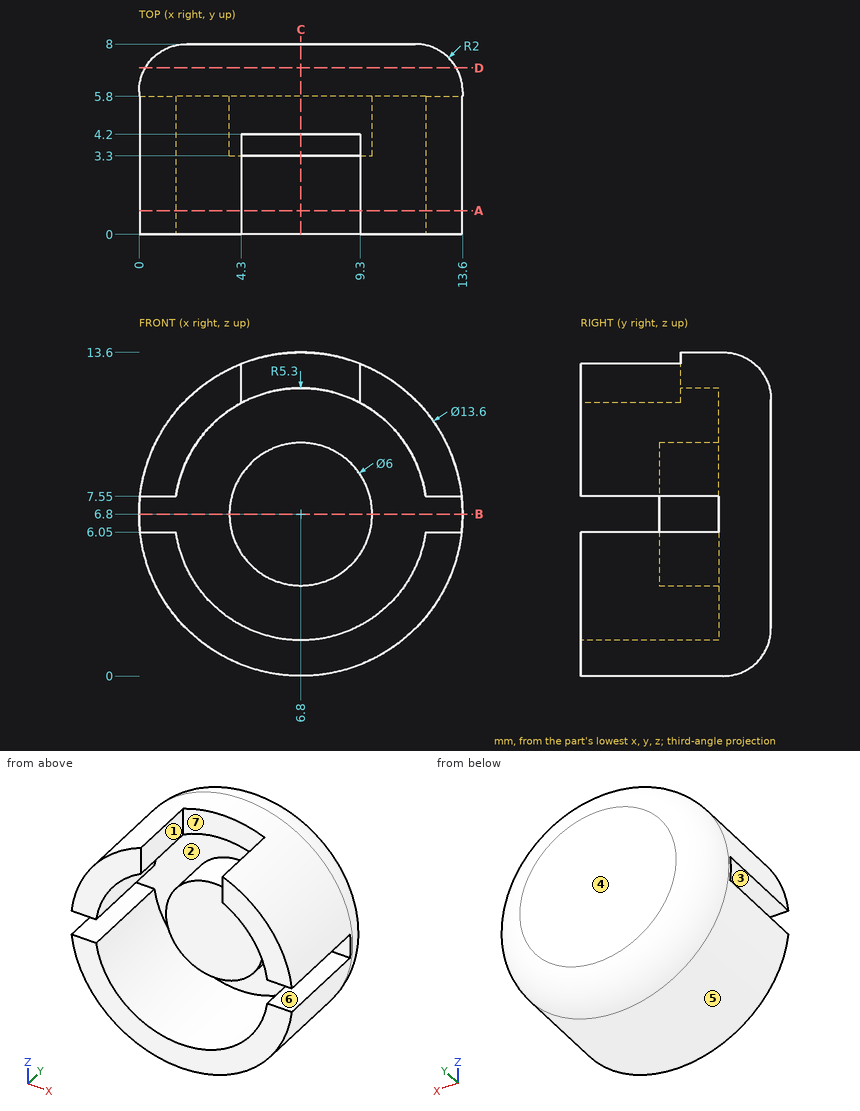
Geometry: see drawing. Coordinates: mm, zero at the bounding-box minimum. A direction names the side the tool comes from. Round coordinates to 2 decimals unless told otherwise and drop trailing zeros. Loops run counter-clockwise (first coordinate to the right, second up) from the corner with the lowest first, then second, coordinate; pieces in that order, holes last. Notation, with made-up numbers: (-32, 33.25) - (17, 33.25) arc R20 ccw to (17, 54.25) - close; hole circle Ø7 at (15, -27.5). An arc over 180 degrees is marked (long way). Use CSV: the item, a comma, the result in double quotes.
Q1. Mould query, pull axis Z, two halves, no side actions, for the marked faces 5, 6 and 7. Classes: pulls with the +Z half, pulls with the -Z half, needs draft (parallel to the pull), parting line crosses it, or undercut.
Reported:
face 5,"parting line crosses it"
face 6,"undercut"
face 7,"needs draft"
Q2. Section query D-D, the plane y = 7. Output: boundary loops of the cut face in (x, z).
Reported:
outline,"circle Ø13.06 at (6.8, 6.8)"
Q3. Reachability of the marked faces 1, 2, 3 and 4 from +Z, -Z, +X, -X, +Y, -Y: full face, straight path, thin tool, end or side. Return the list, or none.
Reported:
face 1,"+Z, -Y"
face 2,"-Y"
face 3,"-X, -Y"
face 4,"+Z, -Z, +X, -X, +Y"
Q4. Pin query (flat end, axial travel): pin 1 Ø1.2 at (x, y) = (13, 2) entering from -Z; pin 2 Ø1 at (x, y) = (2.5, 3.5) entering from -Z; pin 3 Ø0.5 at (x, y) = (0.5, 4) entering from -Z. Return the tip coordinate at first contact, or that it passes through.
Reported:
pin 1,"z = 2.94"
pin 2,"z = 1.16"
pin 3,"z = 3.7"
Q5. Section query C-C, the plane x = 6.8. Output: boundary loops of the cut face in (y, z), then the cut area to 3 significant figures.
Reported:
outline,"(0, 0) - (6, 0) arc R2 ccw to (8, 2) - (8, 11.6) arc R2 ccw to (6, 13.6) - (4.2, 13.6) - (4.2, 12.1) - (5.8, 12.1) - (5.8, 9.8) - (3.3, 9.8) - (3.3, 3.8) - (5.8, 3.8) - (5.8, 1.5) - (0, 1.5) - close"
area,"54.3 mm^2"
Q6. Section query A-A, the plane y = 1. Output: boundary loops of the cut face in (x, z).
Reported:
outline,"(0.04, 6.05) arc R6.8 ccw to (13.56, 6.05) - (12.05, 6.05) arc R5.3 cw to (1.55, 6.05) - close; (0.04, 7.55) - (1.55, 7.55) arc R5.3 cw to (4.3, 11.47) - (4.3, 13.12) arc R6.8 ccw to start; (9.3, 11.47) arc R5.3 cw to (12.05, 7.55) - (13.56, 7.55) arc R6.8 ccw to (9.3, 13.12) - close"
Q7. Ray query, line 1 along X through (y, z) = (4.5, 5.5); line 2 along Y through (x, z) = (10.25, 9). Return the intervals inside material, ascending.
Reported:
line 1,"0.13 to 1.66, 4.1 to 9.5, 11.94 to 13.47"
line 2,"5.8 to 8"
Q8. Section query B-B, the plane z = 6.8. Output: boundary loops of the cut face in (x, y), then the cut area to 3 significant figures.
Reported:
outline,"(0, 5.8) - (3.8, 5.8) - (3.8, 3.3) - (9.8, 3.3) - (9.8, 5.8) - (13.6, 5.8) - (13.6, 6) arc R2 ccw to (11.6, 8) - (2, 8) arc R2 ccw to (0, 6) - close"
area,"43.2 mm^2"
